Job drawing, mm, ordinate dimensions from the low corner. One solid piece. A direction names the side the tool comes from. Give positions to 0.01 mm unless a question says otherwise; leave off trailing zeros. Loops run counter-clockwise (first coordinate to the right, second up) from the corner with the lowest first, then second, coordinate; pieces in that order, holes last. Notation, with made-up numbers: (43.25, -18.75) - (53.25, -18.75) arc R21 ccw to (53.25, 19.25) - close; hole circle Ø5 at (10, -36). An arc over 180 degrees is marked (long way). Use a Markdown table: item, result.
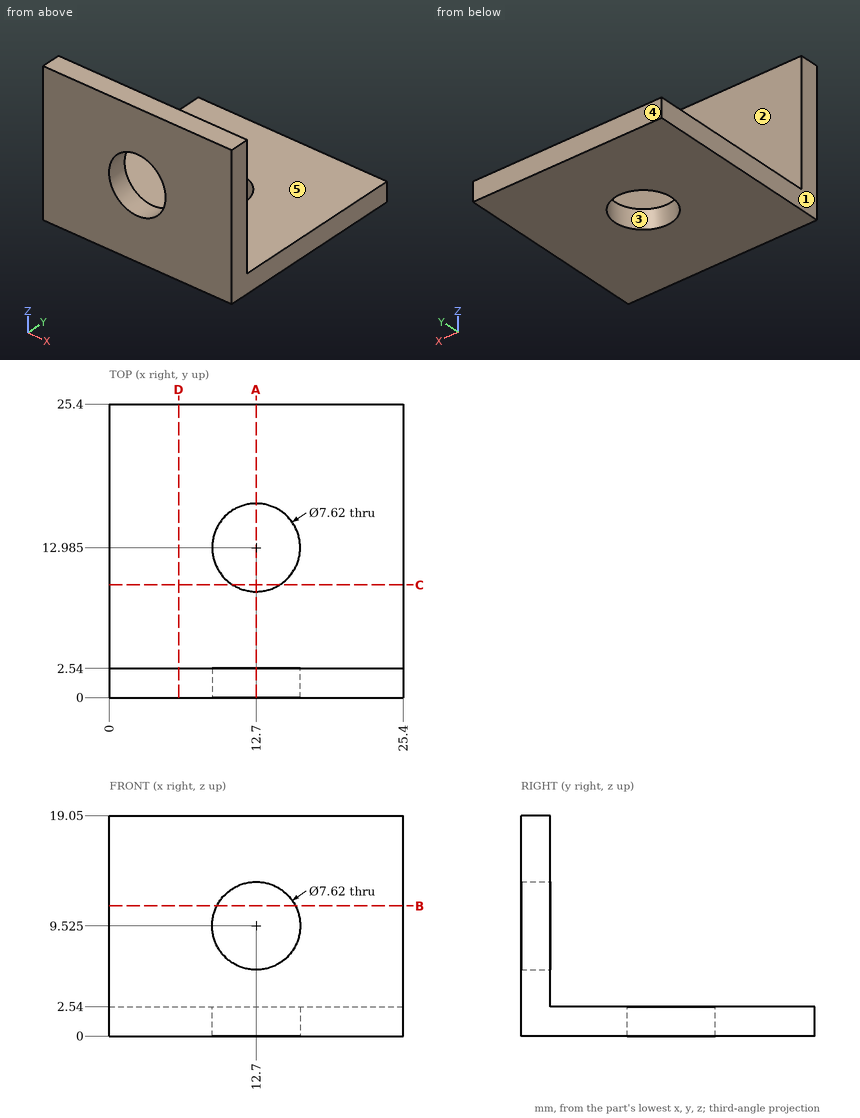
(1) Slice it at D-D, the plane x = 6. Write the cut outline in (y, z).
Computed:
| item | result |
|---|---|
| outline | (0, 0) - (25.4, 0) - (25.4, 2.54) - (2.54, 2.54) - (2.54, 19.05) - (0, 19.05) - close |
(2) 3-axis set-ups, long thin cutter, end or side, ignore diameter. For the marked faces 4 and 5: which of +Z, -Z, +X, -X, +Y, -Y reach the whole face in a straight line?
Computed:
| item | result |
|---|---|
| face 4 | +Z, -Z, +X, -X, +Y |
| face 5 | +Z, +X, -X, +Y |
(3) Drill centre lines: probe 1 along Y at (x, z) = (12.7, 0.95) (3 decimals); probe 2 along Y at (x, z) = (11.75, 15.25). Where is each one in solid material? Low to high. Write a range as [from, to].
Computed:
| item | result |
|---|---|
| probe 1 | [0, 9.175], [16.795, 25.4] |
| probe 2 | [0, 2.54] |
(4) Pin check, flat tips, straight feed: P1, Ø11.5, axis at x = 9, y = 16.5, coming from the +Z side; P2, Ø1.5, axis at y = 6.5, z = 4, coming from the -X side; P3, Ø5, axis at x = 9, z = 14, coming from the +Y side. Stop position of each tip, or through.
Computed:
| item | result |
|---|---|
| P1 | z = 2.54 |
| P2 | through |
| P3 | y = 2.54 |
(5) Slice it at C-C, the plane y = 9.75. Write the cut outline in (x, z), plus the area to 3 significant figures.
Computed:
| item | result |
|---|---|
| outline | (0, 0) - (10.69, 0) - (10.69, 2.54) - (0, 2.54) - close; (14.71, 0) - (25.4, 0) - (25.4, 2.54) - (14.71, 2.54) - close |
| area | 54.3 mm² |
(6) Slice it at A-A, the plane x = 12.7. Write the cut outline in (y, z) (3 decimals).
Computed:
| item | result |
|---|---|
| outline | (0, 0) - (9.175, 0) - (9.175, 2.54) - (2.54, 2.54) - (2.54, 5.715) - (0, 5.715) - close; (0, 13.335) - (2.54, 13.335) - (2.54, 19.05) - (0, 19.05) - close; (16.795, 0) - (25.4, 0) - (25.4, 2.54) - (16.795, 2.54) - close |
(7) Mould opens along X. For the marked faces 1, 2 and 3 say: pulls with the +X half, pulls with the -X half, needs draft (parallel to the pull), parting line crosses it, or undercut.
Computed:
| item | result |
|---|---|
| face 1 | pulls with the -X half |
| face 2 | needs draft |
| face 3 | undercut |
(8) Slice it at B-B, the plane z = 11.25. Write the cut outline in (x, y).
Computed:
| item | result |
|---|---|
| outline | (0, 0) - (9.3, 0) - (9.3, 2.54) - (0, 2.54) - close; (16.1, 0) - (25.4, 0) - (25.4, 2.54) - (16.1, 2.54) - close |
